Geometry: final body of the model. Coordinates: model frame, mm. A direction names the side the tool comes from. Coordinates: 2 decimals unless noted, no trailing zeros. Write each loop counter-clockwise with the first axis right and the second up, starting at its lowest first coordinate (ties: lowest second). Pieces come first, ordered by that corner, then holes.
from build123d import *

# Parameters (mm, degrees)
F0_W     = 32.512
F0_H     = 27.94
F1_DEPTH = 12.7
F2_R     = 1.016
F3_DEPTH = 12.701
F5_DEPTH = 1.651
F6_R     = 1.905
F7_DEPTH = 27.941
F8_R     = 3.556
F9_DEPTH = 18.415


with BuildPart() as f1:
    # F0 (on Right) → F1 (new body)
    with BuildSketch(Plane.YZ):
        with Locations((0, 4.445)):
            Rectangle(F0_W, F0_H)
    extrude(amount=F1_DEPTH)

    # F2 (on face) → F3 (cut, through all)
    with BuildSketch(Plane(origin=(0, 0, 0), x_dir=(0, -1, 0), z_dir=(-1, 0, 0))):
        with Locations((4.7498, 9.525)):
            Circle(F2_R)
        with Locations((-4.7498, 9.525)):
            Circle(F2_R)
    extrude(amount=-F3_DEPTH, mode=Mode.SUBTRACT)

    # F4 (on face) → F5 (cut)
    with BuildSketch(Plane(origin=(0, 0, 0), x_dir=(0, -1, 0), z_dir=(-1, 0, 0))):
        Polygon((-1.96794, 9.682093), (-3.494916, 12.012708), (-6.276777, 11.855615), (-7.53166, 9.367907), (-6.004684, 7.037292), (-3.222823, 7.194385), align=None)
        Polygon((6.142946, 11.938), (3.356654, 11.938), (1.963508, 9.525), (3.356654, 7.112), (6.142946, 7.112), (7.536092, 9.525), align=None)
    extrude(amount=-F5_DEPTH, mode=Mode.SUBTRACT)

    # F6 (on face) → F7 (cut, through all)
    with BuildSketch(Plane.XY.offset(18.415)):
        with Locations((6.35, -9.906)):
            Circle(F6_R)
        with Locations((6.35, 9.906)):
            Circle(F6_R)
    extrude(amount=-F7_DEPTH, mode=Mode.SUBTRACT)

    # F8 (on face) → F9 (cut)
    with BuildSketch(Plane.XY.offset(18.415)):
        with Locations((6.35, 9.906)):
            Circle(F8_R)
        with Locations((6.35, -9.906)):
            Circle(F8_R)
    extrude(amount=-F9_DEPTH, mode=Mode.SUBTRACT)


solid = f1.part
Item 1: Pin query (flat end, axial travel): pin 1 (2 mm diameter, centred on x = 6, y = -10.5, fed in from +Z); pin 2 (5.5 mm diameter, centred on x = 6.35, y = -9.906, fed in from +Z). Return the tip coordinate at first contact, or that it passes through.
Derived:
pin 1: passes through
pin 2: stops at z = 0
Item 2: Material intervals for probe 1 along Y at (x, z) = (6.35, 10.75); probe 2 along X at (y, z) = (10, 4.75); probe 3 along Y at (x, z) = (8.75, 1.5), sorted ascending.
Derived:
probe 1: y = -16.26 to -13.46, -6.35 to 6.35, 13.46 to 16.26
probe 2: x = 0 to 2.8, 9.9 to 12.7
probe 3: y = -16.26 to -12.53, -7.28 to 7.28, 12.53 to 16.26
Item 3: Section D-D, the plane z = 2.25. Output: boundary loops of the cut face in (x, y), plus the area to 3 significant figures.
Derived:
outline: (0, -16.26) - (12.7, -16.26) - (12.7, 16.26) - (0, 16.26) - close; hole circle Ø7.11 at (6.35, -9.91); hole circle Ø7.11 at (6.35, 9.91)
area: 333 mm2
Item 4: Section C-C, the plane y = 9. Output: boundary loops of the cut face in (x, z) (3 decimals), plus the area to 3 significant figures.
Derived:
outline: (0, -9.525) - (4.674, -9.525) - (4.674, 0) - (2.911, 0) - (2.911, 18.415) - (0, 18.415) - close; (8.026, -9.525) - (12.7, -9.525) - (12.7, 18.415) - (9.789, 18.415) - (9.789, 0) - (8.026, 0) - close
area: 196 mm2
Item 5: Set-up query: faces 1 (the flat face through (0.8, 2.7, 10.8)), 2 (the flat face through (8, 8, 0)), 3 (the flat face through (6, 0, 18.415)). Return all of +Z, -Z, +X, -X, +Y, -Y with unobstructed straight access to the full face (end or side cutting, diameter ignored); none if empty.
Derived:
face 1: -X
face 2: +Z
face 3: +Z, +X, -X, +Y, -Y
Item 6: Section B-B, the plane z = 9. Output: boundary loops of the cut face in (x, y), plus the area to 3 significant figures.
Derived:
outline: (0, -16.26) - (12.7, -16.26) - (12.7, -5.62) - (1.65, -5.62) - (1.65, -7.23) - (0, -7.23) - close; (0, -2.27) - (1.65, -2.27) - (1.65, -3.88) - (12.7, -3.88) - (12.7, 3.88) - (1.65, 3.88) - (1.65, 2.31) - (0, 2.31) - close; (0, 7.29) - (1.65, 7.29) - (1.65, 5.62) - (12.7, 5.62) - (12.7, 16.26) - (0, 16.26) - close; hole circle Ø7.11 at (6.35, -9.91); hole circle Ø7.11 at (6.35, 9.91)
area: 279 mm2
Item 7: Section A-A, the plane x = 6.35. Output: boundary loops of the cut face in (y, z) (3 decimals), plus the area to 3 significant figures.
Derived:
outline: (-16.256, -9.525) - (-11.811, -9.525) - (-11.811, 0) - (-13.462, 0) - (-13.462, 18.415) - (-16.256, 18.415) - close; (-8.001, -9.525) - (8.001, -9.525) - (8.001, 0) - (6.35, 0) - (6.35, 18.415) - (-6.35, 18.415) - (-6.35, 0) - (-8.001, 0) - close; (11.811, -9.525) - (16.256, -9.525) - (16.256, 18.415) - (13.462, 18.415) - (13.462, 0) - (11.811, 0) - close; hole circle Ø2.032 at (-4.75, 9.525); hole circle Ø2.032 at (4.75, 9.525)
area: 567 mm2
Item 8: Pull-direction query (Z, two-part tool) for faces 4 (the flat face through (6, 0, -9.525)), 5 (the cylindrical face through (5.937, 8.046, -4.696)), 6 (the flat face through (0.814, 4.633, 7.115)); classes: released by +Z, released by -Z, zero draft, split by the parting line, or undercut.
Derived:
face 4: released by -Z
face 5: zero draft
face 6: undercut
